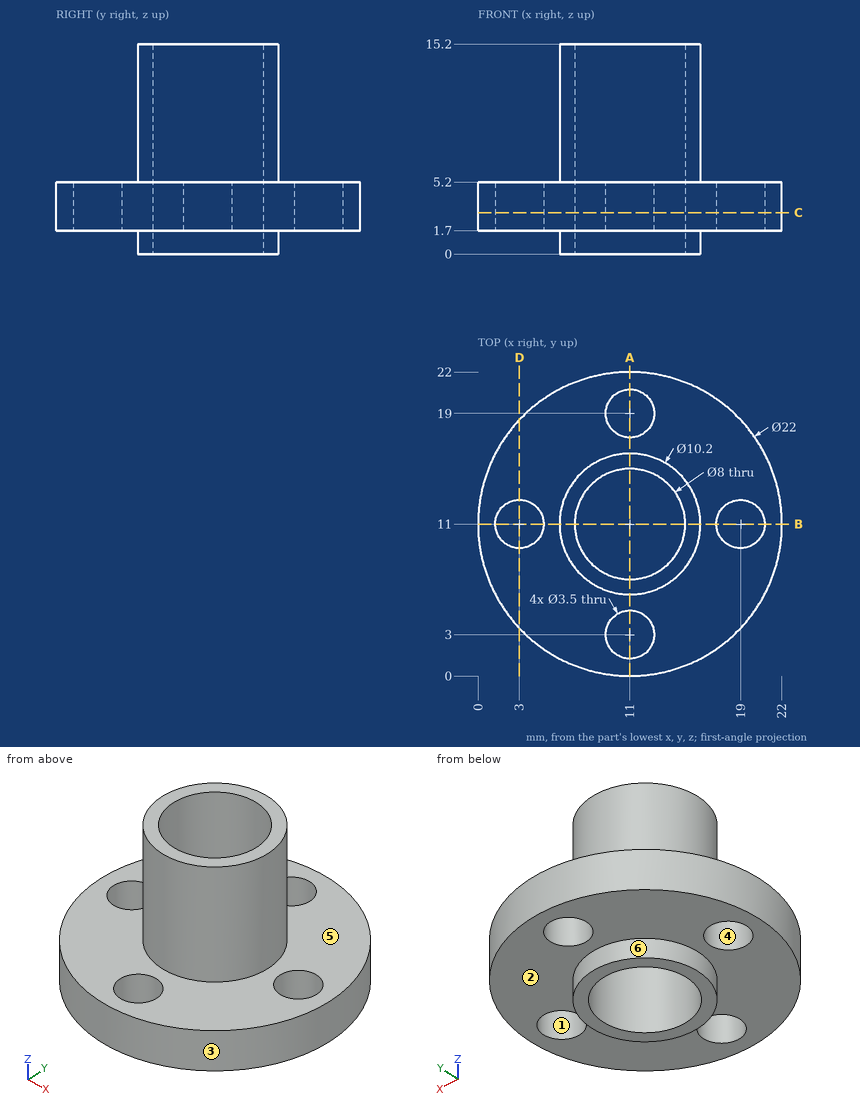
Answer from the drawing. Dimensions are ordinates in mm from the lowest x, y and z of the part. A direction names the side the tool comes from. Round coordinates to 2 decimals unless told otherwise and drop trailing zeros. Write each loop counter-clockwise with the first axis right and the second up, starting at its lowest first coordinate (ties: lowest second). Pieces come first, ordered by that corner, then holes.
1. Straight lines are drawn through the part: L1, parallel to Y at x = 11, z = 3.85; L2, parallel to Y at x = 11, z = 8.5. For each, find the intervals that lie inside material, in ascending order.
2. The part is cut by section A-A, the plane x = 11. Determine the outline of the cut face in (y, z).
3. The part is cut by section D-D, the plane x = 3. Determine the outline of the cut face in (y, z).
4. Given pin 1 Ø1 at (y, z) = (13, 8) entering from +X; pin 2 Ø3 at (x, y) = (11, 3) entering from -Z; pin 3 Ø5 at (y, z) = (17, 10) entering from +X; pin 4 Ø6 at (y, z) = (11.5, 9.5) entering from +X, each flat-ended and moving along its own axis, determine where each tip first touches the part or whether it passes through.
5. Determine the mould class of the marked faces 1, 2 and 3 for opening direction Y: pulls with the +Y half, pulls with the -Y half, needs draft (parallel to the pull), parting line crosses it, or undercut.
6. Which of the six approach directions +Z, -Z, +X, -X, +Y, -Y give full straight-line access (tool end or side, diameter ignored) to the marked faces 4, 5 and 6?
7. The part is cut by section C-C, the plane z = 3. Determine the outline of the cut face in (x, y), then the cut area to 3 significant figures.
Values:
1. L1: y = 0 to 1.25, 4.75 to 7, 15 to 17.25, 20.75 to 22
1. L2: y = 5.9 to 7, 15 to 16.1
2. outline: (0, 1.7) - (1.25, 1.7) - (1.25, 5.2) - (0, 5.2) - close; (4.75, 1.7) - (5.9, 1.7) - (5.9, 0) - (7, 0) - (7, 15.2) - (5.9, 15.2) - (5.9, 5.2) - (4.75, 5.2) - close; (15, 0) - (16.1, 0) - (16.1, 1.7) - (17.25, 1.7) - (17.25, 5.2) - (16.1, 5.2) - (16.1, 15.2) - (15, 15.2) - close; (20.75, 1.7) - (22, 1.7) - (22, 5.2) - (20.75, 5.2) - close
3. outline: (3.45, 1.7) - (9.25, 1.7) - (9.25, 5.2) - (3.45, 5.2) - close; (12.75, 1.7) - (18.55, 1.7) - (18.55, 5.2) - (12.75, 5.2) - close
4. pin 1: stops at x = 15.87
4. pin 2: passes through
4. pin 3: stops at x = 14.71
4. pin 4: stops at x = 16.1
5. face 1: undercut
5. face 2: needs draft
5. face 3: parting line crosses it
6. face 4: +Z, -Z
6. face 5: +Z
6. face 6: -Z
7. outline: circle Ø22 at (11, 11); hole circle Ø3.5 at (3, 11); hole circle Ø8 at (11, 11); hole circle Ø3.5 at (11, 3); hole circle Ø3.5 at (11, 19); hole circle Ø3.5 at (19, 11)
7. area: 291 mm2
